CAD build for the part. Positions are in the model's coordinates, mm. A direction names the side the tool comes from. Give positions to 0.01 mm unless a question says otherwise; leave off trailing zeros. Write each loop counter-clockwise with the first axis right and the second up, starting at its lowest first coordinate (ties: lowest second). Pieces come first, ordered by that corner, then holes. Notation, with made-up numbers: (6, -38.5) -> (21, -38.5) arc R12 cw to (21, -31.5) -> close; hole circle Ø9 at (79.25, 55). An arc over 180 degrees is marked (long way). Answer in a Markdown table with one row per item. Add a question column.
```python
from build123d import *

# Parameters (mm, degrees)
SKETCH_W     = 101
SKETCH_H     = 20
PAD_DEPTH    = 13
SKETCH001_W  = 15
SKETCH001_H  = 20
POCKET_DEPTH = 10
SKETCH002_W  = 20
SKETCH002_H  = 10
PAD001_DEPTH = 8
SKETCH003_W  = 8
SKETCH003_H  = 10
PAD002_DEPTH = 20


with BuildPart() as part:
    # Sketch → Pad (new body)
    with BuildSketch(Plane.XY):
        with Locations((50.5, 10)):
            Rectangle(SKETCH_W, SKETCH_H)
    extrude(amount=PAD_DEPTH)

    # Sketch001 (on Face6 of Pad) → Pocket (cut)
    with BuildSketch(Plane.XY.offset(13)):
        with Locations((12.5, 10)):
            Rectangle(SKETCH001_W, SKETCH001_H)
        with Locations((88.5, 10)):
            Rectangle(SKETCH001_W, SKETCH001_H)
    extrude(amount=-POCKET_DEPTH, mode=Mode.SUBTRACT)

    # Sketch002 (on Face13 of Pocket) → Pad001 (join)
    with BuildSketch(Plane(origin=(0, 0, 0), x_dir=(0, -1, 0), z_dir=(-1, 0, 0))):
        with Locations((-10, 8)):
            Rectangle(SKETCH002_W, SKETCH002_H)
    extrude(amount=PAD001_DEPTH)

    # Sketch003 (on Face14 of Pad001) → Pad002 (join)
    with BuildSketch(Plane.XZ):
        with Locations((-4, 8)):
            Rectangle(SKETCH003_W, SKETCH003_H)
    extrude(amount=PAD002_DEPTH)


solid = part.part
```
Item 1: Slice it at C-C, the plane x = 26. List the corners of the cut face in (y, z).
Item 2: Slice it at B-B, the plane y = 8. List the corners of the cut face in (x, z), then the cut area to 3 significant figures.
Item 3: Which spindle directions (+Z, -Z, +X, -X, +Y, -Y) get a long thin tool onto all of the face, cutting with end or side? Do faces 5 (the face through (98, 10, 13)), 6 (the face through (-4, 0, 3)), 7 (the face through (5, 10, 8)), 8 (the face through (0, -10, 8)), 9 (the face through (-4, -20, 8)). Say none if no direction does.
Item 4: Slice it at A-A, the plane z = 10. List the corners of the cut face in (x, y), then the cut area to 3 significant figures.
Item 5: Probe L1, parallel to X at y = 6.5, z = 12.5; L2, parallel to Y at x = 53.5, z = 9; L3, parallel to X at y = -11, z = 9.25. List the from-to ranges inside material, lowest first. Write a range as from..to.
Item 6: Drop flat-ended pins along their axis: pin 1 Ø3 at (y, z) = (-12, 7.5) entering from +X; pin 2 Ø12 at (x, y) = (85.5, 6) entering from +Z; pin 3 Ø6.5 at (x, y) = (-4.5, -8) entering from -Z; pin 4 Ø3 at (x, z) = (64.5, 6) entering from -Y. Give the stop position or say it passes through.
Item 7: Slice it at D-D, the plane z = 2. List the corners of the cut face in (x, y).
Item 8: Mould opens along X. For faces 1 (the face through (88, 10, 3)), 2 (the face through (47, 20, 6)), 3 (the face through (20, 10, 8)), 4 (the face through (-8, 0, 8)) say: released by +X, released by -X, zero draft, split by the parting line, or undercut.
Answer key:
| question | item | result |
|---|---|---|
| 1 | outline | (0, 0) -> (20, 0) -> (20, 13) -> (0, 13) -> close |
| 2 | outline | (-8, 3) -> (0, 3) -> (0, 0) -> (101, 0) -> (101, 13) -> (96, 13) -> (96, 3) -> (81, 3) -> (81, 13) -> (20, 13) -> (20, 3) -> (5, 3) -> (5, 13) -> (-8, 13) -> close |
| 2 | area | 1,090 mm² |
| 3 | face 5 | +Z, +X, -X, +Y, -Y |
| 3 | face 6 | -Z, -X, +Y, -Y |
| 3 | face 7 | +Z, +Y, -Y |
| 3 | face 8 | +Z, -Z, +X, -Y |
| 3 | face 9 | +Z, -Z, +X, -X, -Y |
| 4 | outline | (-8, -20) -> (0, -20) -> (0, 0) -> (5, 0) -> (5, 20) -> (-8, 20) -> close; (20, 0) -> (81, 0) -> (81, 20) -> (20, 20) -> close; (96, 0) -> (101, 0) -> (101, 20) -> (96, 20) -> close |
| 4 | area | 1,740 mm² |
| 5 | L1 | x = -8..5, 20..81, 96..101 |
| 5 | L2 | y = 0..20 |
| 5 | L3 | x = -8..0 |
| 6 | pin 1 | stops at x = 0 |
| 6 | pin 2 | stops at z = 13 |
| 6 | pin 3 | stops at z = 3 |
| 6 | pin 4 | stops at y = 0 |
| 7 | outline | (0, 0) -> (101, 0) -> (101, 20) -> (0, 20) -> close |
| 8 | face 1 | undercut |
| 8 | face 2 | zero draft |
| 8 | face 3 | undercut |
| 8 | face 4 | released by -X |
